Could you check a few things on this model? Use its own coordinates, in mm. Face numbers are marked on the shaded views. A direction names the side the tool comes from. Coordinates: 2 decimals unless noted, no trailing zeros. Loops run counter-clockwise (first coordinate to the right, second up) from the corner with the lowest first, then second, coordinate; pieces in that order, holes last. Notation, with made-up numbers: (83, 65) - (122, 65) arc R27 ccw to (122, 93) - close; hole circle Ø10 at (60.25, 42). An arc over 180 degrees is marked (long way). One line per item, written item: value. Start each with the question number.
(1) If we section it at B-B on y = 24.5: Write out the boundary of the cut face in (x, z).
(2) If I drill on line 1 along Z through (x, y) = (-41, 44); line 2 along X through (y, z) = (17, -1.7); line 3 along Z through (x, y) = (-5.5, 20), over which ranges is the centre line in solid material (lowest first)? Write a range as from..to.
(3) If we mould it in two halves opening along Z, with no side actions, what happens to the marked faces 3, 4, 5 and 6? For each: pulls with the +Z half, pulls with the -Z half, needs draft (parallel to the pull), parting line crosses it, or undercut.
(4) If we section it at A-A on z = -40.5: Write out the boundary of the cut face in (x, y).
(5) If we section it at D-D on y = 13.5: Write out the boundary of the cut face in (x, z).
(6) On a 3-axis mill with a long thin cutter (end or side, diameter ignored), from which of +Z, -Z, +X, -X, +Y, -Y can I reach the whole of each face in a straight line? I mean the marked faces 1 and 2. Say none if no direction works.
(7) I'm going to push flat-ended pins straight in: P1, Ø3.5, axis at y = 2, z = -37, coming from the -X side; P2, Ø4, axis at x = -13.5, y = 20, coming from the +Z side; P3, Ø8, axis at x = -10.5, z = -51.5, coming from the +Y side; P4, Ø2.5, axis at y = 11, z = -4, coming from the -X side. Where does each tip first touch, or does it pass through?
(8) If we section it at C-C on x = -13: Write out the boundary of the cut face in (y, z), then the cut area to 3 significant figures.
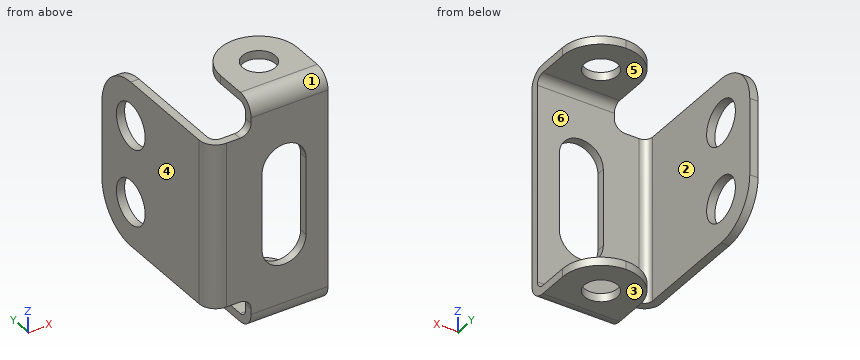
Autodesk Inventor part; units mm, degrees
ref_plane "YZ Plane" through (0, 0, 0) normal (1, 0, 0) x (0, 1, 0)
ref_plane "XZ Plane" through (0, 0, 0) normal (0, 1, 0) x (-1, 0, 0)
ref_plane "XY Plane" through (0, 0, 0) normal (0, 0, 1) x (1, 0, 0)
sketch "Náčrt1" plane through (0, 0, 0) normal (0, 1, 0) x (-1, 0, 0)
  line L0 (0, 0) -> (28, 0)
  line L1 (43, -12) -> (43, -72)
  line L2 (28, -84) -> (0, -84)
  line L3 (0, -84) -> (0, 0)
  line L4 (43, -12) -> (32, -12)
  line L5 (28, -8) -> (28, 0)
  line L6 (28, -84) -> (28, -76)
  line L7 (32, -72) -> (43, -72)
  arc A0 (24, -28) -> (8, -28) centre (16, -28) ccw
  arc A1 (8, -56) -> (24, -56) centre (16, -56) ccw
  line L8 (24, -28) -> (24, -56)
  line L9 (8, -28) -> (8, -56)
  arc A2 (28, -8) -> (32, -12) centre (32, -8) ccw
  arc A3 (32, -72) -> (28, -76) centre (32, -76) ccw
  point P0 (28, -12)
  point P1 (28, -72)
  dimension "d3" = 15
  dimension "d4" = 12
  dimension "d5" = 84
  dimension "d6" = 43
  dimension "d7" = 60
  dimension "d10" = 16
  dimension "d11" = 16
  dimension "d12" = 28
  dimension "d13" = 16
  dimension "d15" = 4
extrude "Deska1" add sketch "Náčrt1" along normal blind 3
sketch "Náčrt2" plane through (0, 0, -3) normal (0, 0, 1) x (1, 0, 0)
  line L0 (-28, 0) -> (0, 0)
  line L1 (0, 0) -> (0, 31)
  line L2 (0, 31) -> (-28, 31)
  line L3 (-28, 31) -> (-28, 0)
edge flange "Obruba1" height 31 angle 90 thickness 3 bend radius 3 thickness toward (0, 0, 1) relief tear relief width 3 relief depth 1.5 corner gap 3 corner form 0 edges at (-14, 3, 0) (-14, 3, -84) wall of the first edge with corners at (-28, 0, -3) (0, 0, -3) (0, 31, -3) (-28, 31, -3)
bend "Ohyb1"
corner "Roh1"
fillet "Zaoblení rohu1" radius 14 4 edges at (-28, 31, -1.5) (0, 31, -1.5) (-28, 31, -82.5) (0, 31, -82.5)
sketch "Náčrt3" plane through (0, 6, -84) normal (0, 0, -1) x (-1, 0, 0)
  line L0 (28, -6) -> (0, -6)
  line L1 (28, 11) -> (28, 0)
  point P0 (14, 11)
  dimension "d27" = 17
  dimension "d28" = 14
hole "Díra1" at (-14, 17, -84) direction (0, 0, 1) diameter 12 depth 3 tip angle 118
sketch "Náčrt4" plane through (-28, 6, 0) normal (0, 0, 1) x (1, 0, 0)
  line L0 (28, -6) -> (0, -6)
  line L1 (28, 11) -> (28, 0)
  point P0 (14, 11)
  dimension "d36" = 17
  dimension "d37" = 14
hole "Díra2" at (-14, 17, 0) direction (0, 0, -1) diameter 12 depth 3 tip angle 118
sketch "Náčrt5" plane through (-40, 0, -12) normal (-1, 0, 0) x (0, -1, 0)
  line L0 (0, -60) -> (0, 0)
  line L1 (0, 0) -> (-60, 0)
  line L2 (-60, 0) -> (-60, -60)
  line L3 (-60, -60) -> (0, -60)
edge flange "Obruba2" height 60 angle 90 thickness 3 bend radius 3 thickness toward (-1, 0, 0) relief tear relief width 3 relief depth 1.5 edges at (-43, 3, -42) wall of the first edge with corners at (-40, 0, -72) (-40, 0, -12) (-40, 60, -12) (-40, 60, -72)
bend "Ohyb2"
corner "Roh2"
fillet "Zaoblení rohu2" radius 16 2 edges at (-41.5, 60, -72) (-41.5, 60, -12)
sketch "Náčrt6" plane through (-43, 6, -72) normal (-1, 0, 0) x (0, 0, 1)
  line L0 (60, -6) -> (0, -6)
  line L1 (0, 0) -> (0, 38)
  point P0 (72, -6)
  point P1 (16, 38)
  dimension "d56" = 44
  dimension "d57" = 16
hole "Díra3" at (-43, 44, -56) direction (1, 0, 0) diameter 16 depth 3 tip angle 118
sketch "Náčrt7" plane through (-43, 6, -72) normal (-1, 0, 0) x (0, 0, 1)
  line L0 (60, -6) -> (0, -6)
  line L1 (60, 38) -> (60, 0)
  point P0 (72, -6)
  point P1 (44, 38)
  dimension "d65" = 44
  dimension "d66" = 16
hole "Díra4" at (-43, 44, -28) direction (1, 0, 0) diameter 16 depth 3 tip angle 118
equation "\"d34\" = Tloušťka"
equation "\"d43\" = Tloušťka"
equation "\"d63\" = Tloušťka"
equation "\"d72\" = Tloušťka"
equation "\"d14\" = Tloušťka"
equation "\"d16\" = ŠířkaVýštipu"
equation "\"d17\" = HloubkaVýštipu"
equation "\"d18\" = MinimálníZbytek"
equation "\"d19\" = PřechodovýPoloměr"
equation "\"d22\" = PoloměrOhybu"
equation "\"d23\" = VelikostRohovéhoVýštipu"
equation "\"d24\" = VelikostMezery"
equation "\"d25\" = VelikostJacobihoPoloměru"
equation "\"d45\" = ŠířkaVýštipu"
equation "\"d46\" = HloubkaVýštipu"
equation "\"d47\" = MinimálníZbytek"
equation "\"d48\" = PřechodovýPoloměr"
equation "\"d51\" = PoloměrOhybu"
equation "\"d52\" = VelikostRohovéhoVýštipu"
equation "\"d53\" = VelikostMezery"
equation "\"d54\" = VelikostJacobihoPoloměru"
equation "\"PoloměrOhybu\" = Tloušťka"
equation "\"ŠířkaVýštipu\" = Tloušťka"
equation "\"HloubkaVýštipu\" = 0.5 * Tloušťka"
equation "\"VelikostRohovéhoVýštipu\" = 4 * Tloušťka"
equation "\"MinimálníZbytek\" = 2 * Tloušťka"
equation "\"PřechodovýPoloměr\" = PoloměrOhybu"
equation "\"VelikostJacobihoPoloměru\" = PoloměrOhybu"
equation "\"VelikostMezery\" = Tloušťka"
properties part number "26886-Vodička_Vojtěch_příklad-3"
Values:
1. outline: (-43, -72) - (-40, -72) - (-40, -12) - (-43, -12) - close; (-25.82, -84) - (-2.18, -84) - (-2.18, -81) - (-25.82, -81) - close; (-25.82, -3) - (-2.18, -3) - (-2.18, 0) - (-25.82, 0) - close
2. line 1: z = -72..-64, -48..-36, -20..-12
2. line 2: x = -28..-20, -8..0
2. line 3: z = -84..-81, -3..0
3. face 3: pulls with the -Z half
3. face 4: needs draft
3. face 5: undercut
3. face 6: undercut
4. outline: (-43, 6) arc R6 ccw to (-37, 0) - (-24, 0) - (-24, 3) - (-37, 3) arc R3 cw to (-40, 6) - (-40, 60) - (-43, 60) - close; (-8, 0) - (0, 0) - (0, 3) - (-8, 3) - close
5. outline: (-43, -72) - (-40, -72) - (-40, -12) - (-43, -12) - close; (-28, -84) - (-18.87, -84) - (-18.87, -81) - (-28, -81) - close; (-28, -3) - (-18.87, -3) - (-18.87, 0) - (-28, 0) - close; (-9.13, -84) - (0, -84) - (0, -81) - (-9.13, -81) - close; (-9.13, -3) - (0, -3) - (0, 0) - (-9.13, 0) - close
6. face 1: +Z, +X, -X, -Y
6. face 2: +Z, -Z, +X, +Y
7. P1: stops at x = -42.56
7. P2: passes through
7. P3: stops at y = 3
7. P4: stops at x = -28
8. outline: (0, -78) arc R6 ccw to (6, -84) - (11.08, -84) - (11.08, -81) - (6, -81) arc R3 cw to (3, -78) - (3, -63.42) - (0, -63.42) - close; (0, -20.58) - (3, -20.58) - (3, -6) arc R3 cw to (6, -3) - (11.08, -3) - (11.08, 0) - (6, 0) arc R6 ccw to (0, -6) - close; (22.92, -84) - (30.96, -84) - (30.96, -81) - (22.92, -81) - close; (22.92, -3) - (30.96, -3) - (30.96, 0) - (22.92, 0) - close
8. area: 209 mm2
